```python
from build123d import *

# Parameters (mm, degrees)
SKETCH1_W           = 22
SKETCH1_H           = 20
BOSS_EXTRUDE1_DEPTH = 400
SKETCH2_R           = 4
CUT_EXTRUDE1_DEPTH  = 23
SKETCH3_W           = 50
SKETCH3_H           = 22
BOSS_EXTRUDE2_DEPTH = 2.2


with BuildPart() as part:
    # Sketch1 → Boss-Extrude1 (new body)
    with BuildSketch(Plane(origin=(0, 0, 0), x_dir=(0, 0, -1), z_dir=(1, 0, 0))):
        Rectangle(SKETCH1_W, SKETCH1_H)
    extrude(amount=BOSS_EXTRUDE1_DEPTH)

    # Sketch2 → Cut-Extrude1 (cut, through all)
    with BuildSketch(Plane.XY.offset(11)):
        with Locations((247, 0)):
            Circle(SKETCH2_R)
    extrude(amount=-CUT_EXTRUDE1_DEPTH, mode=Mode.SUBTRACT)

    # Sketch3 → Boss-Extrude2 (add)
    with BuildSketch(Plane(origin=(0, 10, 0), x_dir=(1, 0, 0), z_dir=(0, 1, 0))):
        with Locations((375, 0)):
            Rectangle(SKETCH3_W, SKETCH3_H)
    extrude(amount=BOSS_EXTRUDE2_DEPTH)


solid = part.part
```
Geometry check sheet. Reference: the model listing, model coordinates, mm. A direction names the side the tool comes from. Coordinates: 2 decimals unless noted, no trailing zeros. Write each loop counter-clockwise with the first axis right and the second up, starting at its lowest first coordinate (ties: lowest second). Pieces come first, ordered by that corner, then holes. Notation, with made-up numbers: M 70,37.25 L 97,37.25 A26 ccw 97,74.25 Z; hole C -8,-23 d1. An arc over 180 degrees is marked long. Use one line per item in the form item = value. Start each with the question number.
1) Section check A-A on y = 0. Enter the section's corners in (x, z), and give its area (3 significant figures).
2) Go/stop test with a flat-tipped pin: pin 1 Ø3 at (x, z) = (75.5, 5) entering from +Y. Record where the tip stops, or that it passes through.
3) Section check B-B on z = -6.5. Enter the section's corners in (x, y).
4) Thickness scan on probe 1 along Y at (x, z) = (247, 0); probe 2 along Y at (x, z) = (61, 0); probe 3 along X at (y, z) = (-1.75, 2.25). Record the ranges inside material, lowest first. Write a range as from..to.
5) Section check C-C on x = 247. Enter the section's corners in (y, z).
6) Set-up check for faces 4 (the flat face through (0, 0, 0)), 5 (the flat face through (173, 10, 0)): record each of +Z, -Z, +X, -X, +Y, -Y from which the full face is reachable in a straight line by a thin tool's end or side.
7) Release check for a two-part mould opening along Y. For faces 1 (the flat face through (375, 12.2, 0)), 2 (the cylindrical face through (243, 0, 0)), 3 (the flat face through (197, -10, 0)) record: pulls with the +Y half, pulls with the -Y half, needs draft (parallel to the pull), parting line crosses it, or undercut.
8) Section check D-D on x = 129.5. Enter the section's corners in (y, z).
Responses:
q1.outline = M 0,-11 L 243,-11 L 243,11 L 0,11 Z; M 251,-11 L 400,-11 L 400,11 L 251,11 Z
q1.area = 8,620 mm2
q2.pin_1 = 10
q3.outline = M 0,-10 L 400,-10 L 400,12.2 L 350,12.2 L 350,10 L 0,10 Z; hole C 247,0 d8
q4.probe_1 = -10..-4, 4..10
q4.probe_2 = -10..10
q4.probe_3 = 0..243.4, 250.6..400
q5.outline = M -10,-11 L -4,-11 L -4,11 L -10,11 Z; M 4,-11 L 10,-11 L 10,11 L 4,11 Z
q6.face_4 = +Z, -Z, -X, +Y, -Y
q6.face_5 = +Z, -Z, -X, +Y
q7.face_1 = pulls with the +Y half
q7.face_2 = undercut
q7.face_3 = pulls with the -Y half
q8.outline = M -10,-11 L 10,-11 L 10,11 L -10,11 Z
